```python
from build123d import *

# Parameters (mm, degrees)
CROQUIS1_W              = 178.587886288
CROQUIS1_H              = 1246.200179681
CROQUIS1_W_2            = 25
CROQUIS1_H_2            = 25
SALIENTE_EXTRUIR2_DEPTH = 285
CROQUIS2_W              = 178.587886288
CROQUIS2_H              = 550.793515283
SALIENTE_EXTRUIR3_DEPTH = 1
CROQUIS5_W              = 25
CROQUIS5_H              = 25
SALIENTE_EXTRUIR4_DEPTH = 2
CROQUIS10_W             = 44.39506519
CROQUIS10_H             = 23.654322963
CROQUIS10_H_2           = 23.654322964
SALIENTE_EXTRUIR5_DEPTH = 1


with BuildPart() as part:
    # Croquis1 → Saliente-Extruir2 (new body)
    with BuildSketch(Plane.XY):
        with Locations((121.784181129, -381.401832721)):
            Rectangle(CROQUIS1_W, CROQUIS1_H)
        with Locations((115.437079382, 174.360479256)):
            Rectangle(CROQUIS1_W_2, CROQUIS1_H_2, mode=Mode.SUBTRACT)
        with Locations((174.990237985, -163.957841157)):
            Rectangle(CROQUIS1_W_2, CROQUIS1_H_2, mode=Mode.SUBTRACT)
        with Locations((115.437079382, 126.027179256)):
            Rectangle(CROQUIS1_W_2, CROQUIS1_H_2, mode=Mode.SUBTRACT)
        with Locations((115.437079382, 77.694179256)):
            Rectangle(CROQUIS1_W_2, CROQUIS1_H_2, mode=Mode.SUBTRACT)
        with Locations((115.437079382, 29.364179256)):
            Rectangle(CROQUIS1_W_2, CROQUIS1_H_2, mode=Mode.SUBTRACT)
        with Locations((115.437079382, -18.965820744)):
            Rectangle(CROQUIS1_W_2, CROQUIS1_H_2, mode=Mode.SUBTRACT)
        with Locations((114.990237985, -67.291541157)):
            Rectangle(CROQUIS1_W_2, CROQUIS1_H_2, mode=Mode.SUBTRACT)
        with Locations((114.990237985, -115.624841157)):
            Rectangle(CROQUIS1_W_2, CROQUIS1_H_2, mode=Mode.SUBTRACT)
        with Locations((114.990237985, -163.957841157)):
            Rectangle(CROQUIS1_W_2, CROQUIS1_H_2, mode=Mode.SUBTRACT)
        with Locations((114.990237985, -212.287841157)):
            Rectangle(CROQUIS1_W_2, CROQUIS1_H_2, mode=Mode.SUBTRACT)
        with Locations((114.990237985, -260.617841157)):
            Rectangle(CROQUIS1_W_2, CROQUIS1_H_2, mode=Mode.SUBTRACT)
        with Locations((174.990237985, -212.287841157)):
            Rectangle(CROQUIS1_W_2, CROQUIS1_H_2, mode=Mode.SUBTRACT)
        with Locations((174.990237985, -260.617841157)):
            Rectangle(CROQUIS1_W_2, CROQUIS1_H_2, mode=Mode.SUBTRACT)
    extrude(amount=-SALIENTE_EXTRUIR2_DEPTH)

    # Croquis2 → Saliente-Extruir3 (add)
    with BuildSketch(Plane(origin=(0, 0, -285), x_dir=(-1, 0, 0), z_dir=(0, 0, -1))):
        with Locations((-121.784181129, -33.698500522)):
            Rectangle(CROQUIS2_W, CROQUIS2_H)
    extrude(amount=-SALIENTE_EXTRUIR3_DEPTH)

    # Croquis5 → Saliente-Extruir4 (add)
    with BuildSketch(Plane.XY):
        Polygon((40.133927115, 241.69825712), (187.776914698, 241.69825712), (211.365707843, 241.69825712), (211.365707843, -1004.501922561), (32.980151612, -1004.501922561), (32.980151612, -301.90284108), (95.791395616, -301.90284108), (95.791395616, 225.342265798), (32.490237985, 225.342265798), (32.490237985, 241.69825712), align=None)
        with Locations((115.723756094, 174.251217897)):
            Rectangle(CROQUIS5_W, CROQUIS5_H, mode=Mode.SUBTRACT)
        with Locations((175.276914698, -164.067102515)):
            Rectangle(CROQUIS5_W, CROQUIS5_H, mode=Mode.SUBTRACT)
        with Locations((115.723756094, 125.917917897)):
            Rectangle(CROQUIS5_W, CROQUIS5_H, mode=Mode.SUBTRACT)
        with Locations((115.723756094, 77.584917897)):
            Rectangle(CROQUIS5_W, CROQUIS5_H, mode=Mode.SUBTRACT)
        with Locations((115.723756094, 29.254917897)):
            Rectangle(CROQUIS5_W, CROQUIS5_H, mode=Mode.SUBTRACT)
        with Locations((115.723756094, -19.075082103)):
            Rectangle(CROQUIS5_W, CROQUIS5_H, mode=Mode.SUBTRACT)
        with Locations((115.276914698, -67.400802515)):
            Rectangle(CROQUIS5_W, CROQUIS5_H, mode=Mode.SUBTRACT)
        with Locations((115.276914698, -115.734102515)):
            Rectangle(CROQUIS5_W, CROQUIS5_H, mode=Mode.SUBTRACT)
        with Locations((115.276914698, -164.067102515)):
            Rectangle(CROQUIS5_W, CROQUIS5_H, mode=Mode.SUBTRACT)
        with Locations((115.276914698, -212.397102515)):
            Rectangle(CROQUIS5_W, CROQUIS5_H, mode=Mode.SUBTRACT)
        with Locations((115.276914698, -260.727102515)):
            Rectangle(CROQUIS5_W, CROQUIS5_H, mode=Mode.SUBTRACT)
        with Locations((175.276914698, -212.397102515)):
            Rectangle(CROQUIS5_W, CROQUIS5_H, mode=Mode.SUBTRACT)
        with Locations((175.276914698, -260.727102515)):
            Rectangle(CROQUIS5_W, CROQUIS5_H, mode=Mode.SUBTRACT)
    extrude(amount=SALIENTE_EXTRUIR4_DEPTH)

    # Croquis10 → Saliente-Extruir5 (add)
    with BuildSketch(Plane.XY):
        with Locations((62.970480914, 172.960872416)):
            Rectangle(CROQUIS10_W, CROQUIS10_H)
        with Locations((64.427271282, 75.386790193)):
            Rectangle(CROQUIS10_W, CROQUIS10_H_2)
        with Locations((64.427271282, -20.708896845)):
            Rectangle(CROQUIS10_W, CROQUIS10_H)
        with Locations((64.427271282, -69.495937956)):
            Rectangle(CROQUIS10_W, CROQUIS10_H)
        with Locations((64.427271282, -118.282979068)):
            Rectangle(CROQUIS10_W, CROQUIS10_H)
        with Locations((62.948876097, -164.113229809)):
            Rectangle(CROQUIS10_W, CROQUIS10_H)
        with Locations((62.948876097, -209.94348055)):
            Rectangle(CROQUIS10_W, CROQUIS10_H)
        with Locations((64.427271282, 28.078144267)):
            Rectangle(CROQUIS10_W, CROQUIS10_H)
        with Locations((64.427271282, 124.173831305)):
            Rectangle(CROQUIS10_W, CROQUIS10_H)
        with Locations((64.427271282, -261.687312031)):
            Rectangle(CROQUIS10_W, CROQUIS10_H_2)
    extrude(amount=SALIENTE_EXTRUIR5_DEPTH)


solid = part.part
```
Check sheet for the modelled part. Datum: model origin and axes. Units: mm. Give positions to 0.01 mm unless a question says otherwise; leave off trailing zeros. Answer in a Markdown table with one row per item.
1) Thickness scan on L1, parallel to X at y = -162.5, z = -220.5; L2, parallel to Y at x = 181.5, z = -65; L3, parallel to X at y = 31, z = -26.5. Record the ranges inside material, lowest first. Write a range as [from, to].
Filled sheet:
| item | result |
|---|---|
| L1 | x = [32.49, 102.49], [127.49, 162.49], [187.49, 211.08] |
| L2 | y = [-1004.5, -273.12], [-248.12, -224.79], [-199.79, -176.46], [-151.46, 241.7] |
| L3 | x = [32.49, 102.94], [127.94, 211.08] |
2) Cross-section at A-A, the plane z = -45.5. Count the separate pieces of the cut face and the enclosed holes in it, plus the area to 3 significant figures.
Filled sheet:
| item | result |
|---|---|
| separate pieces | 1 |
| enclosed holes | 13 |
| area | 214,000 mm2 |
3) Gauge pin test, flat ends, axial feed: P1, Ø1.6, axis at y = -209.5, z = 1, coming from the -X side; P2, Ø3, axis at y = -253.5, z = -242, coming from the +X side; P3, Ø0.5, axis at y = 72, z = 0.5, coming from the -X side. Record the tip position at first contact, or that the pin passes through.
Filled sheet:
| item | result |
|---|---|
| P1 | stops at x = 40.75 |
| P2 | stops at x = 211.08 |
| P3 | stops at x = 42.23 |
4) Release check for a two-part mould opening along X. For faces 1 (the flat face through (115, -67, -284)), 2 (the flat face through (64, -21, 1)), 3 (the flat face through (32.49, -390, -144)) record: +X half, -X half, draft (parallel to the pull), parting line (faces both ways), or undercut.
Filled sheet:
| item | result |
|---|---|
| face 1 | undercut |
| face 2 | draft |
| face 3 | -X half |
